```python
from build123d import *

# Parameters (mm, degrees)
CROQUIS1_R              = 18.2625
SALIENTE_EXTRUIR1_DEPTH = 3
CROQUIS2_R              = 15.5
SALIENTE_EXTRUIR2_DEPTH = 120
CROQUIS3_R              = 14.75
CORTAR_EXTRUIR1_DEPTH   = 102


with BuildPart() as part:
    # Croquis1 → Saliente-Extruir1 (new body)
    with BuildSketch(Plane(origin=(0, 0, 0), x_dir=(1, 0, 0), z_dir=(0, 1, 0))):
        with Locations(Location((0, 0, 0), (0, 0, 270))):
            Circle(CROQUIS1_R)
    extrude(amount=SALIENTE_EXTRUIR1_DEPTH)

    # Croquis2 → Saliente-Extruir2 (add)
    with BuildSketch(Plane(origin=(0, 3, 0), x_dir=(1, 0, 0), z_dir=(0, 1, 0))):
        with Locations(Location((0, 0, 0), (0, 0, 270))):
            Circle(CROQUIS2_R)
    extrude(amount=SALIENTE_EXTRUIR2_DEPTH)

    # Croquis3 → Cortar-Extruir1 (cut)
    with BuildSketch(Plane.XZ):
        with Locations(Location((0, 0, 0), (0, 0, 270))):
            Circle(CROQUIS3_R)
    extrude(amount=-CORTAR_EXTRUIR1_DEPTH, mode=Mode.SUBTRACT)

    # Croquis4 → Cortar-Revolución3 (revolve, cut)
    with BuildSketch(Plane.XY):
        Polygon((0, 102), (-14.75, 102), (-13.2, 123), (0, 123), align=None)
    revolve(axis=Axis((0, 123, 0), (0, -1, 0)), mode=Mode.SUBTRACT)


solid = part.part
```
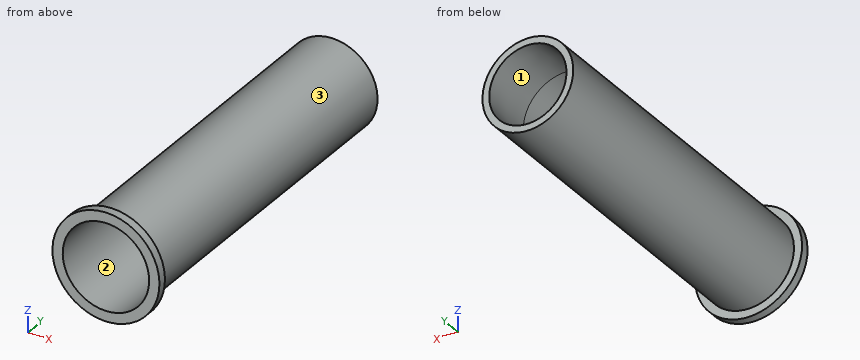
Input: part model. Units: mm. Frame: model coordinates. Face numbers are marked on the shaded views. Round coordinates to 2 decimals unless told otherwise and drop trailing zeros. Loops run counter-clockwise (first coordinate to the right, second up) from the corner with the lowest first, then second, coordinate; pieces in that order, holes last. Notation, with made-up numbers: (63.25, -20) -> (105.25, -20) arc R20 cw to (105.25, -1) -> close; hole circle Ø3 at (37, 57). An arc over 180 degrees is marked (long way). Use one line per item in the form item = value. Start each with the question number.
Item 1: Material intervals for L1, parallel to X at y = 53, z = 0; L2, parallel to Z at x = 2, y = 35.5; L3, parallel to Y at x = -15.5, z = -9, sorted ascending. Write a range as from..to.
Item 2: Section query C-C on y = 76.5. Return the cut outline in (x, z), then the cut area to 3 significant figures.
Item 3: Section query A-A on z = 0. Return the cut outline in (x, y).
Item 4: Mould query, pull axis Z, two halves, no side actions, for the marked faces 1, 2 and 3. Classes: pulls with the +Z half, pulls with the -Z half, needs draft (parallel to the pull), parting line crosses it, or undercut.
Item 5: Contact query for flat-ended pins moving along their axis: pin 1 Ø5 at (x, y) = (-5.5, 33) entering from -Z; pin 2 Ø3 at (x, y) = (7, 69) entering from -Z; pin 3 Ø10 at (y, z) = (88.5, 11) entering from +X. Output: stop coordinate, or through.
Item 6: Section query B-B on x = 0. Return the cut outline in (y, z), then the cut area to 3 significant figures.
Ans:
q1.L1 = -15.5..-14.75, 14.75..15.5
q1.L2 = -15.37..-14.61, 14.61..15.37
q1.L3 = 0..3
q2.outline = circle Ø31 at (0, 0); hole circle Ø29.5 at (0, 0)
q2.area = 71.3 mm^2
q3.outline = (-18.26, 0) -> (-14.75, 0) -> (-14.75, 102) -> (-13.2, 123) -> (-15.5, 123) -> (-15.5, 3) -> (-18.26, 3) -> close; (13.2, 123) -> (14.75, 102) -> (14.75, 0) -> (18.26, 0) -> (18.26, 3) -> (15.5, 3) -> (15.5, 123) -> close
q4.face_1 = undercut
q4.face_2 = undercut
q4.face_3 = parting line crosses it
q5.pin_1 = -15.21
q5.pin_2 = -14.49
q5.pin_3 = 14.29
q6.outline = (0, -18.26) -> (3, -18.26) -> (3, -15.5) -> (123, -15.5) -> (123, -13.2) -> (102, -14.75) -> (0, -14.75) -> close; (0, 14.75) -> (102, 14.75) -> (123, 13.2) -> (123, 15.5) -> (3, 15.5) -> (3, 18.26) -> (0, 18.26) -> close
q6.area = 234 mm^2
